Geometry check sheet. Reference: drawing and pictorial views, mm from the part's lowest x, y, z. Round coordinates to 2 decimals unless told otherwise and drop trailing zeros. Write each loop counter-clockwise with the first axis right and the second up, starting at its lowest first coordinate (ties: lowest second). Pieces come first, ordered by that corner, then holes. Notation, with made-up numbers: M 24.25,68 L 28.25,68 A27 ccw 28.25,91 Z; hole C 87.25,87.5 d6. An arc over 180 degrees is marked long. Answer in a Markdown table with one row per item.
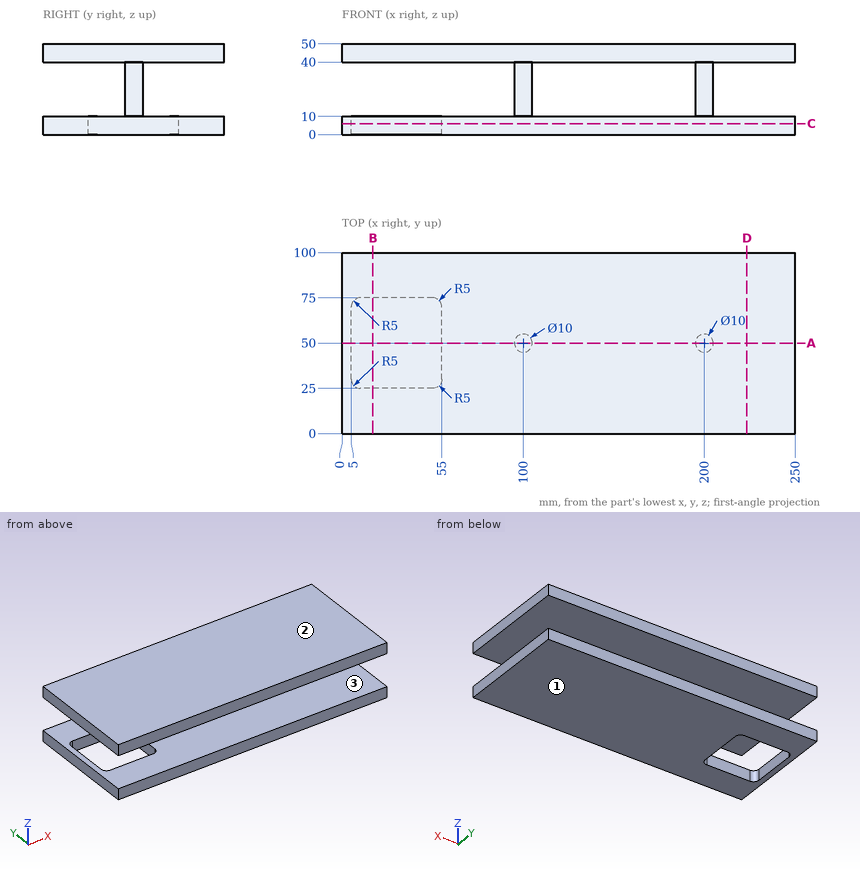
1. Scan lines: L1, parallel to Z at x = 110, y = 86.5; L2, parallel to X at y = 46.5, z = 32; L3, parallel to Z at x = 49, y = 70. Record each from-to range of solid material in increasing order.
Found:
| item | result |
|---|---|
| L1 | z = 0 to 10, 40 to 50 |
| L2 | x = 96.43 to 103.57, 196.43 to 203.57 |
| L3 | z = 40 to 50 |
2. Section check A-A, the plane y = 50. Record the cut outline in (x, z), and give its area (3 significant figures).
Found:
| item | result |
|---|---|
| outline | M 0,0 L 5,0 L 5,10 L 0,10 Z; M 0,40 L 95,40 L 95,10 L 55,10 L 55,0 L 250,0 L 250,10 L 205,10 L 205,40 L 250,40 L 250,50 L 0,50 Z; hole M 105,10 L 195,10 L 195,40 L 105,40 Z |
| area | 5,100 mm2 |
3. Section check D-D, the plane x = 223.5. Record the cut outline in (y, z).
Found:
| item | result |
|---|---|
| outline | M 0,0 L 100,0 L 100,10 L 0,10 Z; M 0,40 L 100,40 L 100,50 L 0,50 Z |
4. Section check C-C, the plane z = 6. Record the cut outline in (x, y).
Found:
| item | result |
|---|---|
| outline | M 0,0 L 250,0 L 250,100 L 0,100 Z; hole M 5,30 A5 ccw 10,25 L 50,25 A5 ccw 55,30 L 55,70 A5 ccw 50,75 L 10,75 A5 ccw 5,70 Z |
5. Section check B-B, the plane x = 17. Record the cut outline in (y, z), and give its area (3 significant figures).
Found:
| item | result |
|---|---|
| outline | M 0,0 L 25,0 L 25,10 L 0,10 Z; M 0,40 L 100,40 L 100,50 L 0,50 Z; M 75,0 L 100,0 L 100,10 L 75,10 Z |
| area | 1,500 mm2 |
6. Draft check along Z on the marked faces 1, 2 and 3. Enter one of: +Z half, -Z half, draft (parallel to the pull), parting line (faces both ways), or undercut.
Found:
| item | result |
|---|---|
| face 1 | -Z half |
| face 2 | +Z half |
| face 3 | undercut |
